from build123d import *

# Parameters (mm, degrees)
BOSS_EXTRUDE1_DEPTH = 135
SKETCH3_W           = 40
SKETCH3_H           = 31
BOSS_EXTRUDE2_DEPTH = 20
CHAMFER1_SIZE       = 30


with BuildPart() as part:
    # Sketch2 → Boss-Extrude1 (new body)
    with BuildSketch(Plane.XY):
        with BuildLine():
            Line((114.838111964, -46.094555434), (77.599019601, -24.594555434))
            ThreePointArc((77.599019601, -24.594555434), (76.081381511, -24.394754589), (74.866968793, -25.326606241))
            Line((74.866968793, -25.326606241), (59.366968793, -52.173393759))
            ThreePointArc((59.366968793, -52.173393759), (59.167167948, -53.691031849), (60.099019601, -54.905444566))
            Line((60.099019601, -54.905444566), (97.338111964, -76.405444566))
            Line((97.338111964, -76.405444566), (114.838111964, -46.094555434))
        make_face()
    extrude(amount=BOSS_EXTRUDE1_DEPTH)

    # Sketch3 → Boss-Extrude2 (add)
    with BuildSketch(Plane(origin=(67.116968793, -38.75, 0), x_dir=(0, 0, 1), z_dir=(-0.866025404, 0.5, 0))):
        with Locations((115, 0)):
            Rectangle(SKETCH3_W, SKETCH3_H)
    extrude(amount=BOSS_EXTRUDE2_DEPTH)

    # Chamfer1
    chamfer1_edges = [part.edges().sort_by_distance(p)[0] for p in [
        (106.088111964, -61.25, 135),
    ]]
    chamfer(chamfer1_edges, length=CHAMFER1_SIZE)


solid = part.part
The model under review builds one solid part; all positions refer to its coordinate system, in mm. A direction names the side the tool comes from. Give positions to 0.01 mm unless a question says otherwise; leave off trailing zeros. Write each loop counter-clockwise with the first axis right and the second up, starting at its lowest first coordinate (ties: lowest second). Pieces come first, ordered by that corner, then holes.
1. Add section A-A, the plane z = 102.5. Write out the cut boundary in (x, y), plus the area to 3 significant figures.
2. Add section B-B, the plane y = -37.5. Write out the cut boundary in (x, z), plus the area to 3 significant figures.
3. Draft analysis for pull direction X (two halves, no side actions). For faces 1 (the cylindrical face through (76.1, -24.39, 66.55)), 2 (the flat face through (87, -50, 0)), 3 (the flat face through (93.157, -54.067, 119.79)), state which applies: +X half, -X half, draft (parallel to the pull), parting line (faces both ways), or undercut.
4. Add section C-C, the plane x = 79. Write out the cut boundary in (y, z), plus the area to 3 significant figures.
5. Tool access review of faces 4 (the cylindrical face through (59.16, -53.67, 66.55)), 5 (the flat face through (67.225, -38.562, 46.835)): name each direction out of +Z, -Z, +X, -X, +Y, -Y from which nothing blocks a thin tool from reaching the whole face with its end or side.
6. Wall thickness on L1, parallel to Z at x = 67, y = -35; L2, parallel to Z at x = 84, y = -68; L3, parallel to X at y = -73, z = 36.5: over which ranges is each line inside the solid? List them lowest first.
7. For P1, Ø6, axis at y = -30, z = 89.5, coming from the -X side; P2, Ø8, axis at x = 99.5, y = -61, coming from the -Z side; P3, Ø8, axis at y = -42, z = 49.5, coming from the +X side; P4, Ø10, axis at x = 61.5, y = -37, coming from the -Z side, all flat-tipped, find the tip position at first contact; note any pin that passes through.
8. Add section D-D, the plane z = 22. Write out the cut boundary in (x, y).
Worked answers:
1. outline: (42.05, -42.17) - (59.37, -52.17) arc R2 ccw to (60.1, -54.91) - (97.34, -76.41) - (114.84, -46.09) - (77.6, -24.59) arc R2 ccw to (74.87, -25.33) - (57.55, -15.33) - close
1. area: 2,190 mm2
2. outline: (44.74, 95) - (67.84, 95) - (67.84, 0) - (99.95, 0) - (99.95, 122.19) - (85.16, 135) - (44.74, 135) - close
2. area: 5,160 mm2
3. face 1: undercut
3. face 2: draft
3. face 3: +X half
4. outline: (-65.82, 0) - (-25.4, 0) - (-25.4, 135) - (-48.17, 135) - (-65.82, 126.18) - close
4. area: 5,380 mm2
5. face 4: +Z, -Z, -X
5. face 5: -Z, -X, +Y
6. L1: z = 95 to 135
6. L2: z = 0 to 120.75
6. L3: x = 91.44 to 99.3
7. P1: stops at x = 70.44
7. P2: stops at z = 0
7. P3: stops at x = 114.67
7. P4: stops at z = 95
8. outline: (59.37, -52.17) arc R2 ccw to (60.1, -54.91) - (97.34, -76.41) - (114.84, -46.09) - (77.6, -24.59) arc R2 ccw to (74.87, -25.33) - close
